Source: CAD feature listing. Evaluate the final solid. Frame: model axes, mm. A direction names the side the tool comes from. Give positions to 0.01 mm unless a question says otherwise; leave off trailing zeros. Write each loop counter-clockwise with the first axis right and the second up, starting at its lowest first coordinate (ties: lowest second). Pieces come first, ordered by that corner, then holes. Notation, with made-up numbers: M -10,-8.5 L 49,-8.5 A26 cw 49,6.5 Z; hole C -39,30.25 d4. An arc over 180 degrees is marked long. Use CSV: the item, a comma, the result in double quotes. Start each with the question number.
from build123d import *

# Parameters (mm, degrees)
F0_W          = 33.12
F0_H          = 20.57
F1_DEPTH      = 0.63
F3_DEPTH      = 17.69
F4_W          = 19.23
F4_H          = 12.16
F5_DEPTH      = 15.21
F6_R          = 2.065
F7_DEPTH      = 19.2
F7_DEPTH_BACK = 16.95


with BuildPart() as f1:
    # F0 (on Front) → F1 (new body, symmetric)
    with BuildSketch(Plane.XZ):
        Rectangle(F0_W, F0_H)
    extrude(amount=F1_DEPTH, both=True)

    # F2 (on face) → F3 (join)
    with BuildSketch(Plane.XZ.offset(0.63)):
        Polygon((16.56, 0), (9.705, 7.38), (-9.705, 7.38), (-16.56, 0), (-9.705, -7.38), (9.705, -7.38), align=None)
    extrude(amount=F3_DEPTH)

    # F4 (on face) → F5 (cut)
    with BuildSketch(Plane(origin=(0, 0.63, 0), x_dir=(-1, 0, 0), z_dir=(0, 1, 0))):
        Rectangle(F4_W, F4_H)
        Polygon((15.56, 0), (9.615, 6.08), (9.615, -6.08), align=None)
        Polygon((-9.615, -6.08), (-9.615, 6.08), (-15.56, 0), align=None)
    extrude(amount=-F5_DEPTH, mode=Mode.SUBTRACT)

    # F6 (on face) → F7 (join, two sides)
    with BuildSketch(Plane.XZ.offset(18.32)) as f7_sk:
        with Locations((-9.705, 0)):
            Circle(F6_R)
        with Locations((9.705, 0)):
            Circle(F6_R)
    extrude(amount=F7_DEPTH)
    extrude(f7_sk.sketch, amount=-F7_DEPTH_BACK)


solid = f1.part
Item 1: Set-up query: faces 5 (the flat face through (13.18, -9.35, 3.64)), 6 (the flat face through (0, -0.63, -8)), 7 (the cylindrical face through (-7.735, -8.067, 0.62)), 8 (the flat face through (-13.085, -9.351, 3.742)), 9 (the cylindrical face through (11.675, -27.786, 0.62)). Return all of +Z, -Z, +X, -X, +Y, -Y with unobstructed straight access to the full face (end or side cutting, diameter ignored); none if empty.
Item 2: Section A-A (y = -3). Return the cut outline in (x, z) (3 decimals).
Item 3: Material intervals for probe 1 along Z at (x, y) = (-0.5, -2); probe 2 along Z at (x, y) = (-7.5, -17); probe 3 along Z at (x, y) = (-11.5, -8), sorted ascending.
Item 4: Section B-B (x = -11). Return the cut outline in (y, z) (3 decimals), plus the area to 3 significant figures.
Item 5: Section C-C (y = -33.5). Return the cut outline in (x, z) (3 decimals).
Item 6: Pull-direction query (X, two-part tool) for faces 1 (the flat face through (-13.18, -9.35, -3.64)), 2 (the flat face through (13.085, -9.351, -3.742)), 3 (the flat face through (0, 0.63, 7)), 4 (the flat face through (10, -1.37, 0)); classes: released by +X, released by -X, zero draft, split by the parting line, or undercut.
Item 7: Contact query for flat-ended pins moving along their axis: pin 1 Ø2 at (y, z) = (-33.5, 1) entering from +X; pin 2 Ø10 at (y, z) = (-12, -2.5) entering from +X; pin 3 Ø12 at (x, y) = (-1, -10.5) entering from -Z. Output: stop coordinate, or through.
Item 8: Section D-D (z = -3.75). Return the cut outline in (x, y).
Output values:
1,face 5,"+Z, +X, -Y"
1,face 6,"-Z, -Y"
1,face 7,"+Y"
1,face 8,"+Z, -X, -Y"
1,face 9,"-Y"
2,outline,"M -16.56,0 L -9.705,-7.38 L 9.705,-7.38 L 16.56,0 L 9.705,7.38 L -9.705,7.38 Z; C -9.705,0 d4.13; C 9.705,0 d4.13; hole M -15.56,0 L -9.615,-6.08 L 9.615,-6.08 L 15.56,0 L 9.615,6.08 L -9.615,6.08 Z"
3,probe 1,"z = -7.38 to -6.08, 6.08 to 7.38"
3,probe 2,"z = -7.38 to 7.38"
3,probe 3,"z = -5.45 to -4.15, -1.02 to 1.02, 4.15 to 5.45"
4,outline,"M -37.52,-1.608 L -18.32,-1.608 L -18.32,-5.986 L -0.63,-5.986 L -0.63,-10.285 L 0.63,-10.285 L 0.63,-4.664 L -14.58,-4.664 L -14.58,-1.608 L -1.37,-1.608 L -1.37,1.608 L -14.58,1.608 L -14.58,4.664 L 0.63,4.664 L 0.63,10.285 L -0.63,10.285 L -0.63,5.986 L -18.32,5.986 L -18.32,1.608 L -37.52,1.608 Z"
4,area,"200 mm2"
5,outline,"C -9.705,0 d4.13; C 9.705,0 d4.13"
6,face 1,"released by -X"
6,face 2,"released by +X"
6,face 3,"zero draft"
6,face 4,"undercut"
7,pin 1,"stops at x = 11.77"
7,pin 2,"stops at x = 16.56"
7,pin 3,"stops at z = -7.38"
8,outline,"M -16.56,-0.63 L -13.08,-0.63 L -13.08,-18.32 L 13.08,-18.32 L 13.08,-0.63 L 16.56,-0.63 L 16.56,0.63 L 11.89,0.63 L 11.89,-14.58 L -11.89,-14.58 L -11.89,0.63 L -16.56,0.63 Z"
